```python
from build123d import *

# Parameters (mm, degrees)
F0_R     = 19.4658001659
F1_DEPTH = 25.4
F2_T     = -2.54
F3_DEPTH = 25.4
F4_DEPTH = 25.4
F5_R     = 5.08


with BuildPart() as f1:
    # F0 (on Front) → F1 (new body)
    with BuildSketch(Plane.XZ):
        with Locations((-37.8019884229, 38.6502295732)):
            Circle(F0_R)
    extrude(amount=F1_DEPTH)

    # F2
    f2_openings = [f1.faces().sort_by_distance(p)[0] for p in [
        (-37.801988, -25.4, 38.65023),
    ]]
    offset(amount=F2_T, openings=f2_openings)

    # F3 (add): a face of the model
    f3_faces = [f1.faces().sort_by_distance(p)[0] for p in [
        (-56.7172126168, -25.4, 38.6502295732),
    ]]
    extrude(f3_faces, amount=-F3_DEPTH)

    # F4 (add): a face of the model
    f4_faces = [f1.faces().sort_by_distance(p)[0] for p in [
        (-56.7172126168, -25.4, 38.6502295732),
    ]]
    extrude(f4_faces, amount=F4_DEPTH)

    # F5
    f5_edges = [f1.edges().sort_by_distance(p)[0] for p in [
        (-57.267789, 0, 38.65023),
    ]]
    fillet(f5_edges, radius=F5_R)


solid = f1.part
```
Check sheet for the modelled part. Datum: model origin and axes. Units: mm. A direction names the side the tool comes from. Round coordinates to 2 decimals unless told otherwise and drop trailing zeros. Order: outer loops, then holes, each group sorted by start corner. A loop starts at its lowest first (then second) coordinate and runs counter-clockwise, first axis right, second up.
1) Go/stop test with flat-tipped pins: pin 1 Ø6 at (y, z) = (-17, 33) entering from -X; pin 2 Ø1 at (x, z) = (-32.5, 34) entering from -Y; pin 3 Ø4 at (x, z) = (-36, 48.5) entering from +Y; pin 4 Ø3 at (y, z) = (-39.5, 52.5) entering from -X. Record where each tip stops, or that it passes through.
2) Scan lines: line 1 (X direction, y = -42.5, z = 38.5); line 2 (Z direction, x = -38.5, y = -26.5); line 3 (X direction, y = -24, z = 25). Record each from-to range of solid material in increasing order.
3) Section check A-A (y = -14.5). Record the boundary of the cut face in (x, z), and give its area (3 significant figures).
4) Tool access check on faces 1 (the flat face through (-44, -50.8, 55)), 2 (the cylindrical face through (-54.71, -26.33, 39.39)). Record the directions out of +Z, -Z, +X, -X, +Y, -Y that give a thin tool (end or side, any length) a straight path to the whole face; none if there is none.
5) Mould release check, pull along Z, two halves, no side actions. Record for faces 3 (the cylindrical face through (-19.821, -27.62, 31.195)), 4 (the flat face through (-38, 0, 39)), 5 (the flat face through (-38, -2.54, 39)): +Z half, -Z half, draft (parallel to the pull), parting line (faces both ways), or undercut.
Result:
1. pin 1: stops at x = -57.09
1. pin 2: stops at y = -2.54
1. pin 3: stops at y = 0
1. pin 4: stops at x = -52.85
2. line 1: x = -57.27 to -54.73, -20.88 to -18.34
2. line 2: z = 19.2 to 21.74, 55.56 to 58.1
2. line 3: x = -51.68 to -47.81, -27.79 to -23.92
3. outline: circle Ø38.93 at (-37.8, 38.65); hole circle Ø33.85 at (-37.8, 38.65)
3. area: 290 mm2
4. face 1: +Z, -Z, +X, -X, -Y
4. face 2: -Y
5. face 3: parting line
5. face 4: draft
5. face 5: undercut
